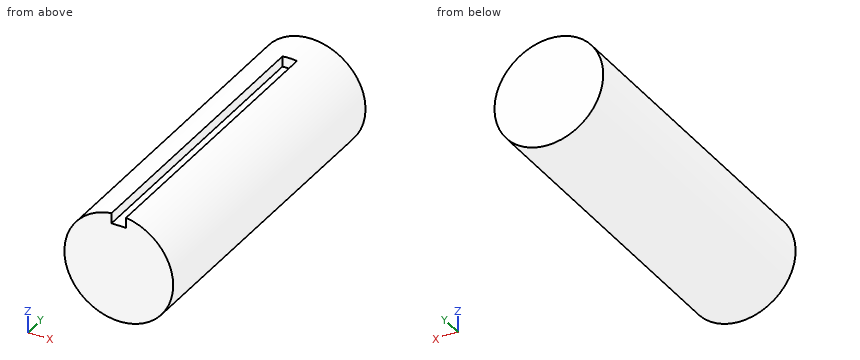
Solid Edge part; units mm, degrees
sketch "Sketch1" plane through (0, 0, 0) normal (0, -1, 0) x (1, 0, 0)
  circle A0 centre (0, 0) radius 15
extrude "Protrusion1" add sketch "Sketch1" against normal blind 90
sketch "Sketch2" plane through (0, 0, 0) normal (0, -1, 0) x (1, 0, 0)
  line L0 (-2, 16.5083) -> (2, 16.5083)
  line L1 (2, 16.5083) -> (2, 12)
  line L2 (2, 12) -> (-2, 12)
  line L3 (-2, 12) -> (-2, 16.5083)
  dimension "D1" = 2
extrude "ExtrudedCutout_1" cut sketch "Sketch2" against normal blind 80
properties part number "1"
Part model, mm, in its own coordinate system. Round coordinates to 2 decimals unless told otherwise and drop trailing zeros. Write each loop counter-clockwise with the first axis right and the second up, starting at its lowest first coordinate (ties: lowest second). Pieces come first, ordered by that corner, then holes. Notation, with made-up numbers: (-2.5, 46.25) -> (22.5, 46.25) arc R19 cw to (22.5, 77.25) -> close; hole circle Ø7 at (62.25, 7.25). An arc over 180 degrees is marked (long way). Return JSON: item names as keys, results as strings. Group by question number.
Q1. Saw through at B-B on y = 61. Write the cut outline in (x, z), plus the area to 3 significant figures.
Q2. Pin check, flat tips, straight feed: pin 1 (6 mm diameter, centred on x = -9, y = 51, fed in from +Z); pin 2 (6 mm diameter, centred on y = 14.5, z = -4.5, fed in from +X); pin 3 (2 mm diameter, centred on y = 31.5, z = 11, fed in from -X). Stop position of each tip, or through.
Q3. Saw through at C-C on z = 6.25. Write the cut outline in (x, y), plus the area to 3 significant figures.
Q4. Probe L1, parallel to Z at x = 0.5, y = 4; L2, parallel to X at y = 35.5, z = 13.5; L3, parallel to Z at x = 1.25, y = 5.5. List the from-to ranges inside material, lowest first. Write a range as [from, to].
Q5. Saw through at A-A on x = 0. Write the cut outline in (y, z), plus the area to 3 significant figures.
Answer:
{
 "1": {"outline": "(-2, 12) -> (-2, 14.87) arc R15 ccw (long way) to (2, 14.87) -> (2, 12) -> close", "area": "695 mm2"},
 "2": {"pin 1": "z = 13.75", "pin 2": "x = 14.92", "pin 3": "x = -11.18"},
 "3": {"outline": "(-13.64, 0) -> (13.64, 0) -> (13.64, 90) -> (-13.64, 90) -> close", "area": "2,450 mm2"},
 "4": {"L1": "[-14.99, 12]", "L2": "[-6.54, -2], [2, 6.54]", "L3": "[-14.95, 12]"},
 "5": {"outline": "(0, -15) -> (90, -15) -> (90, 15) -> (80, 15) -> (80, 12) -> (0, 12) -> close", "area": "2,460 mm2"}
}
